Work out the finished part from the listing and answer in its coordinate system (mm). A direction names the side the tool comes from. Round coordinates to 2 decimals unless told otherwise and drop trailing zeros. Order: outer loops, then holes, each group sorted by start corner. A loop starts at its lowest first (then second) coordinate and runs counter-clockwise, first axis right, second up. Notation, with made-up numbers: (45, 25.25) - (91, 25.25) arc R9 ccw to (91, 34.25) - close; hole circle Ø8 at (67, -18.5). An arc over 180 degrees is marked (long way). Answer in a Markdown table with one row per item.
Autodesk Inventor part; units mm, degrees
ref_plane "YZ Plane" through (0, 0, 0) normal (1, 0, 0) x (0, 1, 0)
ref_plane "XZ Plane" through (0, 0, 0) normal (0, 1, 0) x (-1, 0, 0)
ref_plane "XY Plane" through (0, 0, 0) normal (0, 0, 1) x (1, 0, 0)
sketch "スケッチ1" plane through (0, 0, 0) normal (0, 1, 0) x (-1, 0, 0)
  line L0 (0, 0) -> (45.1, 0)
  line L1 (45.1, 0) -> (45.1, -24.1)
  line L2 (45.1, -24.1) -> (0, -24.1)
  line L3 (0, -24.1) -> (0, 0)
  dimension "d0" = 45.1
  dimension "d1" = 24.1
extrude "押し出し1" add sketch "スケッチ1" along normal blind 14
sketch "スケッチ2" plane through (0, 14, 0) normal (0, 1, 0) x (1, 0, 0)
  line L0 (-45.1, 0) -> (0, 0)
  line L1 (-28, 0) -> (-28, 24.1)
  line L2 (0, 24.1) -> (-45.1, 24.1)
  point P0 (-28, 4)
  point P1 (-28, 20.1)
  dimension "d4" = 4
  dimension "d5" = 4
hole "穴1" at (-28, 14, -4) at (-28, 14, -20.1) direction (0, -1, 0) diameter 3 end through all counterbore diameter 6 counterbore depth 3.3
sketch "スケッチ3" plane through (0, 0, 0) normal (0, -1, 0) x (1, 0, 0)
  circle A0 centre (-28, -20.1) radius 1.5
  line L0 (-28, -20.1) -> (-28, 0)
  circle A1 centre (-28, -20.1) radius 3
  circle A2 centre (-28, -4) radius 1.5
  point P0 (0, 0)
hole "穴2" at (-28, 0, -20.1) at (-28, 0, -4) direction (0, 1, 0) diameter 3 end through all counterbore diameter 6 counterbore depth 3.3
sketch "スケッチ4" plane through (0, 0, 0) normal (0, -1, 0) x (1, 0, 0)
  line L0 (0, 0) -> (-45.1, 0)
  line L1 (-16, 0) -> (-16, -23.8904)
  line L2 (0, -24.1) -> (-45.1, -24.1)
  line L3 (-21.5, -24.1) -> (-21.5, 0)
  point P0 (-16, -4.5)
  point P1 (-21.5, -19.6)
  dimension "d20" = 4.5
  dimension "d21" = 4.5
hole "穴3" at (-16, 0, -4.5) at (-21.5, 0, -19.6) direction (0, 1, 0) diameter 2.3 end through all
sketch "スケッチ5" plane through (-45.1, 0, -24.1) normal (-1, 0, 0) x (0, 0, 1)
  line L0 (0, 14) -> (24.1, 14)
  line L1 (12.05, 14) -> (12.05, 0)
  circle A0 centre (12.05, 7) radius 3.05
  circle A1 centre (12.05, 7) radius 2.5
  point P0 (24.1, 0)
  dimension "d40" = 6.1
  dimension "d41" = 5
sketch "スケッチ6" plane through (-45.1, 0, 0) normal (0, 0, 1) x (1, 0, 0)
  line L0 (11.25, 13.7757) -> (11.25, 0)
  line L1 (0, 0) -> (0, 14)
  line L2 (45.1, 0) -> (0, 0)
  line L3 (45.1, 14) -> (0, 14)
  line L4 (33.85, 14) -> (33.85, 0)
  line L5 (45.1, 0) -> (45.1, 14)
  point P0 (11.25, 6)
  point P1 (33.85, 7.75)
  dimension "d29" = 11.25
  dimension "d30" = 6
  dimension "d31" = 11.25
  dimension "d32" = 6.25
hole "穴4" at (-11.25, 7.75, 0) at (-33.85, 6, 0) direction (0, 0, -1) diameter 4.1 depth 5.8 tip angle 118
extrude "押し出し2" add sketch "スケッチ5" along normal blind 1 contours A0 L1 A1 | L1 A1 A0
sketch "スケッチ8" plane through (-45.1, 0, -24.1) normal (-1, 0, 0) x (0, 0, 1)
  circle A0 centre (12.05, 7) radius 3.05
  point P0 (24.1, 0)
hole "穴5" at (-45.1, 7, -12.05) direction (1, 0, 0) diameter 5 depth 20
properties part number "KOGANEI_BDA10X15"
1) Find the intervals of material crossed by probe 1 along Z at (x, y) = (-28, 1.4); probe 2 along Y at (x, z) = (-30, -12.05); probe 3 along Y at (x, z) = (-34, -3), in increasing order. Write a range as from..to.
Filled in:
| item | result |
|---|---|
| probe 1 | z = -24.1..-23.1, -17.1..-7, -1..0 |
| probe 2 | y = 0..4.5, 9.5..14 |
| probe 3 | y = 0..3.96, 8.04..14 |
2) Find section D-D, the plane z = -19.6. Give the vertices of the cut face in (x, y), then the cut area to 3 significant figures.
Filled in:
| item | result |
|---|---|
| outline | (-45.1, 0) - (-30.96, 0) - (-30.96, 3.3) - (-29.41, 3.3) - (-29.41, 10.7) - (-30.96, 10.7) - (-30.96, 14) - (-45.1, 14) - close; (-26.59, 3.3) - (-25.04, 3.3) - (-25.04, 0) - (-22.65, 0) - (-22.65, 14) - (-25.04, 14) - (-25.04, 10.7) - (-26.59, 10.7) - close; (-20.35, 0) - (0, 0) - (0, 14) - (-20.35, 14) - close |
| area | 539 mm^2 |
3) Each of these flat-tipped pins is pushed along its axis until it touches: pin 1 (2.5 mm diameter, centred on x = -28, z = -4, fed in from -Y); pin 2 (5.5 mm diameter, centred on x = -28, z = -4, fed in from +Y); pin 3 (1.5 mm diameter, centred on y = 6, z = -12, fed in from -X); pin 4 (8 mm diameter, centred on y = 11, z = -18.5, fed in from -X). Where does it stop, or does it pass through?
Filled in:
| item | result |
|---|---|
| pin 1 | passes through |
| pin 2 | stops at y = 10.7 |
| pin 3 | stops at x = -25.1 |
| pin 4 | stops at x = -45.1 |
4) The mould has two halves that part along X. Classify faces 5 (the face through (-26.7, 10.7, -18.8)), 6 (the face through (-35.45, 9.44, -12.59)), 7 (the face through (-45.1, 5, -9)): released by +X, released by -X, zero draft, split by the parting line, or undercut.
Filled in:
| item | result |
|---|---|
| face 5 | undercut |
| face 6 | zero draft |
| face 7 | released by -X |
5) Find section A-A, the plane x = -28. Give the number of separate pieces and of enclosed holes in the cut face, then the cut area to 3 significant figures.
Filled in:
| item | result |
|---|---|
| separate pieces | 3 |
| enclosed holes | 1 |
| area | 194 mm^2 |
6) Find section C-C, the plane x = -16. Give the vertices of the cut face in (y, z), then the cut area to 3 significant figures.
Filled in:
| item | result |
|---|---|
| outline | (0, -24.1) - (14, -24.1) - (14, -5.65) - (0, -5.65) - close; (0, -3.35) - (14, -3.35) - (14, 0) - (0, 0) - close |
| area | 305 mm^2 |
7) Find section B-B, the plane y = 2.75. Give the vertices of the cut face in (x, z).
Filled in:
| item | result |
|---|---|
| outline | (-45.1, -24.1) - (0, -24.1) - (0, 0) - (-45.1, 0) - close; hole circle Ø6 at (-28, -20.1); hole circle Ø6 at (-28, -4); hole circle Ø2.3 at (-21.5, -19.6); hole circle Ø2.3 at (-16, -4.5) |
8) Which of the six approach directions +Z, -Z, +X, -X, +Y, -Y give full straight-line access (tool end or side, diameter ignored) to faces 1 (the face through (-35.883, 6.267, -2.941)), 2 (the face through (-45.593, 9.977, -12.711)), 3 (the face through (-28.1, 12.3, -23.1)), 4 (the face through (-26.85, 1.67, -22.87))?
Filled in:
| item | result |
|---|---|
| face 1 | +Z |
| face 2 | -X |
| face 3 | +Y |
| face 4 | -Y |
